Work out the finished part from the listing and answer in its coordinate system (mm). Round coordinates to 2 decimals unless told otherwise and drop trailing zeros. Order: outer loops, then holes, each group sorted by start corner. A loop starts at its lowest first (then second) coordinate and runs counter-clockwise, first axis right, second up. Notation, with made-up numbers: (75, 86.25) - (102, 86.25) arc R27 cw to (102, 121.25) - close; hole circle Ø6 at (86, 0.25). An arc over 180 degrees is marked (long way). Answer in a Markdown table with one row per item.
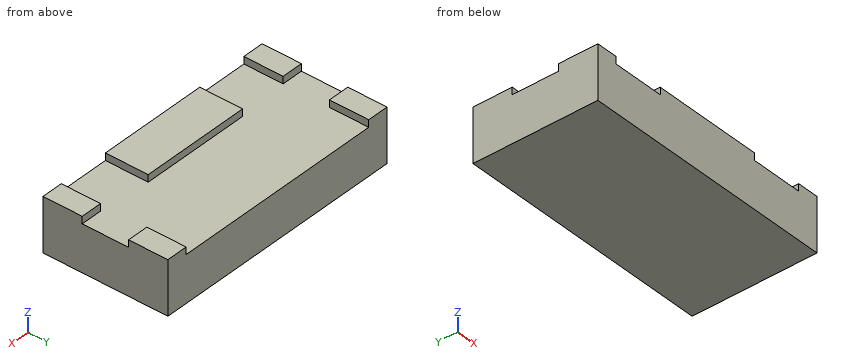
from build123d import *

# Parameters (mm, degrees)
BOX024_W     = 3.1
BOX024_H     = 1.2
BOX024_DEPTH = 0.2
BOX023_W     = 0.6
BOX023_H     = 1.1
BOX023_DEPTH = 0.2
BOX022_W     = 0.6
BOX022_H     = 1.1
BOX022_DEPTH = 0.2
BOX021_W     = 0.6
BOX021_H     = 1.1
BOX021_DEPTH = 0.2
BOX020_W     = 0.6
BOX020_H     = 1.1
BOX020_DEPTH = 0.2
BOX025_W     = 7.2
BOX025_H     = 3.5
BOX025_DEPTH = 0.2
BOX_W        = 7.2
BOX_H        = 3.5
BOX_DEPTH    = 1.5


with BuildPart() as cube024:
    # Box024 → Box024 (new body)
    with BuildSketch(Plane(origin=(2.05, 0, 1.3), x_dir=(1, 0, 0), z_dir=(0, 0, 1))):
        with Locations((1.55, 0.6)):
            Rectangle(BOX024_W, BOX024_H)
    extrude(amount=BOX024_DEPTH)


with BuildPart() as cube023:
    # Box023 → Box023 (new body)
    with BuildSketch(Plane(origin=(0, 2.4, 1.3), x_dir=(1, 0, 0), z_dir=(0, 0, 1))):
        with Locations((0.3, 0.55)):
            Rectangle(BOX023_W, BOX023_H)
    extrude(amount=BOX023_DEPTH)


with BuildPart() as cube022:
    # Box022 → Box022 (new body)
    with BuildSketch(Plane.XY.offset(1.3)):
        with Locations((0.3, 0.55)):
            Rectangle(BOX022_W, BOX022_H)
    extrude(amount=BOX022_DEPTH)


with BuildPart() as cube021:
    # Box021 → Box021 (new body)
    with BuildSketch(Plane(origin=(6.6, 2.4, 1.3), x_dir=(1, 0, 0), z_dir=(0, 0, 1))):
        with Locations((0.3, 0.55)):
            Rectangle(BOX021_W, BOX021_H)
    extrude(amount=BOX021_DEPTH)


with BuildPart() as cube020:
    # Box020 → Box020 (new body)
    with BuildSketch(Plane(origin=(6.6, 0, 1.3), x_dir=(1, 0, 0), z_dir=(0, 0, 1))):
        with Locations((0.3, 0.55)):
            Rectangle(BOX020_W, BOX020_H)
    extrude(amount=BOX020_DEPTH)


with BuildPart() as silver_top001:
    # Box025 → Box025 (new body)
    with BuildSketch(Plane.XY.offset(1.3)):
        with Locations((3.6, 1.75)):
            Rectangle(BOX025_W, BOX025_H)
    extrude(amount=BOX025_DEPTH)

    # Cut005: cut Cube020
    add(cube020.part, mode=Mode.SUBTRACT)

    # Cut009: cut Cube021
    add(cube021.part, mode=Mode.SUBTRACT)

    # Cut006: cut Cube022
    add(cube022.part, mode=Mode.SUBTRACT)

    # Cut008: cut Cube023
    add(cube023.part, mode=Mode.SUBTRACT)

    # Cut007: cut Cube024
    add(cube024.part, mode=Mode.SUBTRACT)


with BuildPart() as plastic_body:
    # Box → Box (new body)
    with BuildSketch(Plane.XY):
        with Locations((3.6, 1.75)):
            Rectangle(BOX_W, BOX_H)
    extrude(amount=BOX_DEPTH)

    # Cut010: cut Silver Top001
    add(silver_top001.part, mode=Mode.SUBTRACT)


solid = plastic_body.part
1) Find the intervals of material crossed by probe 1 along Z at (x, y) = (5.5, 1); probe 2 along Y at (x, z) = (4.25, 1.35), in increasing order. Write a range as from..to.
Filled in:
| item | result |
|---|---|
| probe 1 | z = 0..1.3 |
| probe 2 | y = 0..1.2 |
2) Find section B-B, the plane y = 2.8. Give the vertices of the cut face in (x, z).
Filled in:
| item | result |
|---|---|
| outline | (0, 0) - (7.2, 0) - (7.2, 1.5) - (6.6, 1.5) - (6.6, 1.3) - (0.6, 1.3) - (0.6, 1.5) - (0, 1.5) - close |
3) Find section D-D, the plane y = 1.45. Give the vertices of the cut face in (x, z), then the cut area to 3 significant figures.
Filled in:
| item | result |
|---|---|
| outline | (0, 0) - (7.2, 0) - (7.2, 1.3) - (0, 1.3) - close |
| area | 9.36 mm^2 |
4) Find section A-A, the plane x = 4.75. Give the vertices of the cut face in (y, z).
Filled in:
| item | result |
|---|---|
| outline | (0, 0) - (3.5, 0) - (3.5, 1.3) - (1.2, 1.3) - (1.2, 1.5) - (0, 1.5) - close |
5) Find section C-C, the plane y = 0.9. Give the vertices of the cut face in (x, z).
Filled in:
| item | result |
|---|---|
| outline | (0, 0) - (7.2, 0) - (7.2, 1.5) - (6.6, 1.5) - (6.6, 1.3) - (5.15, 1.3) - (5.15, 1.5) - (2.05, 1.5) - (2.05, 1.3) - (0.6, 1.3) - (0.6, 1.5) - (0, 1.5) - close |
